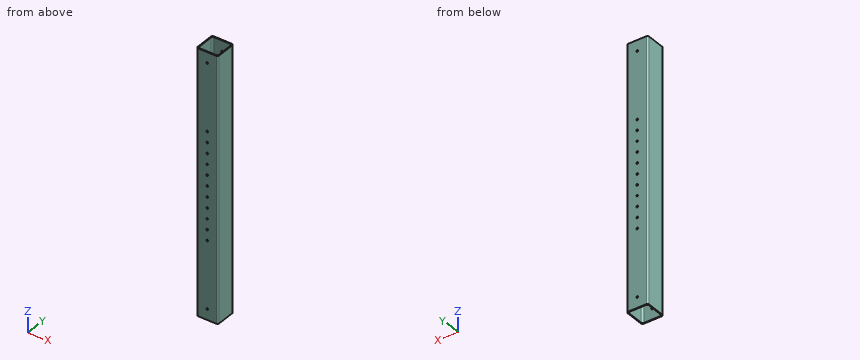
from build123d import *

# Parameters (mm, degrees)
SKETCH1_W           = 70
SKETCH1_H           = 70
SKETCH1_W_2         = 64
SKETCH1_H_2         = 64
BOSS_EXTRUDE1_DEPTH = 860
FILLET1_R           = 5
SKETCH2_R           = 3
CUT_EXTRUDE1_DEPTH  = 70
SKETCH3_R           = 3
CUT_EXTRUDE2_DEPTH  = 173
LPATTERN1_COUNT     = 6
LPATTERN1_PITCH     = 35
LPATTERN1_COL_COUNT = 6
LPATTERN1_COL_PITCH = 35


with BuildPart() as part:
    # Sketch1 → Boss-Extrude1 (new body)
    with BuildSketch(Plane.XY):
        with Locations((35, 35)):
            Rectangle(SKETCH1_W, SKETCH1_H)
        with Locations((35, 35)):
            Rectangle(SKETCH1_W_2, SKETCH1_H_2, mode=Mode.SUBTRACT)
    extrude(amount=BOSS_EXTRUDE1_DEPTH)

    # Fillet1
    fillet1_edges = [part.edges().sort_by_distance(p)[0] for p in [
        (3, 67, 430),
        (3, 3, 430),
        (67, 3, 430),
        (67, 67, 430),
        (0, 70, 430),
        (70, 70, 430),
        (70, 0, 430),
        (0, 0, 430),
    ]]
    fillet(fillet1_edges, radius=FILLET1_R)

    # Sketch2 → Cut-Extrude1 (cut)
    with BuildSketch(Plane(origin=(0, 70, 0), x_dir=(1, 0, 0), z_dir=(0, 1, 0))):
        with Locations(Location((35, -825, 0), (0, 0, 270))):
            Circle(SKETCH2_R)
        with Locations(Location((35, -35, 0), (0, 0, 270))):
            Circle(SKETCH2_R)
    extrude(amount=-CUT_EXTRUDE1_DEPTH, mode=Mode.SUBTRACT)

    # Sketch3 → Cut-Extrude2 (cut)
    with BuildSketch(Plane.XZ):
        with Locations(Location((35, 430, 0), (0, 0, 270))):
            Circle(SKETCH3_R)
    cut_extrude2 = extrude(amount=-CUT_EXTRUDE2_DEPTH, mode=Mode.SUBTRACT)

    # LPattern1: Cut-Extrude2 ×6
    with Locations(*[(0, 0, -i * LPATTERN1_PITCH) for i in range(1, LPATTERN1_COUNT)]):
        add(cut_extrude2, mode=Mode.SUBTRACT)

    # LPattern1 col: Cut-Extrude2 ×6
    with Locations(*[(0, 0, i * LPATTERN1_COL_PITCH) for i in range(1, LPATTERN1_COL_COUNT)]):
        add(cut_extrude2, mode=Mode.SUBTRACT)


solid = part.part
Geometry check sheet. Reference: the model listing, model coordinates, mm. Give positions to 0.01 mm unless a question says otherwise; leave off trailing zeros. Loops run counter-clockwise (first coordinate to the right, second up) from the corner with the lowest first, then second, coordinate; pieces in that order, holes last.
(1) Depth check by flat-ended pin: pin 1 Ø5 at (x, z) = (35, 570) entering from +Y. Enter the tip coordinate at first touch or a pass-through.
From the geometry:
pin 1: passes through
(2) Section check A-A on z = 713.5. Record the cut outline in (x, y), then the cut area to 3 significant figures.
From the geometry:
outline: (0, 5) arc R5 ccw to (5, 0) - (65, 0) arc R5 ccw to (70, 5) - (70, 65) arc R5 ccw to (65, 70) - (5, 70) arc R5 ccw to (0, 65) - close; hole (3, 8) arc R5 ccw to (8, 3) - (62, 3) arc R5 ccw to (67, 8) - (67, 62) arc R5 ccw to (62, 67) - (8, 67) arc R5 ccw to (3, 62) - close
area: 804 mm2
(3) Thickness scan on L1, parallel to Y at x = 42.5, z = 452.5; L2, parallel to Y at x = 4, z = 506. Record the ranges inside material, lowest first.
From the geometry:
L1: y = 0 to 3, 67 to 70
L2: y = 0.1 to 5, 65 to 69.9
